Could you check a few things on this drawing? It's one solid part, dimensions in mm from its lowest x, y, z. Round coordinates to 2 decimals unless told otherwise and drop trailing zeros. Write each loop counter-clockwise with the first axis right and the second up, starting at its lowest first coordinate (ties: lowest second). Pieces come first, ordered by that corner, then holes. Notation, with made-up numbers: (2, 30.25) -> (37, 30.25) arc R20 cw to (37, 67.25) -> close; hole circle Ø8 at (-37, 68.25). An arc over 180 degrees is marked (long way). Answer in a Markdown table with one row per item. Add a question column.
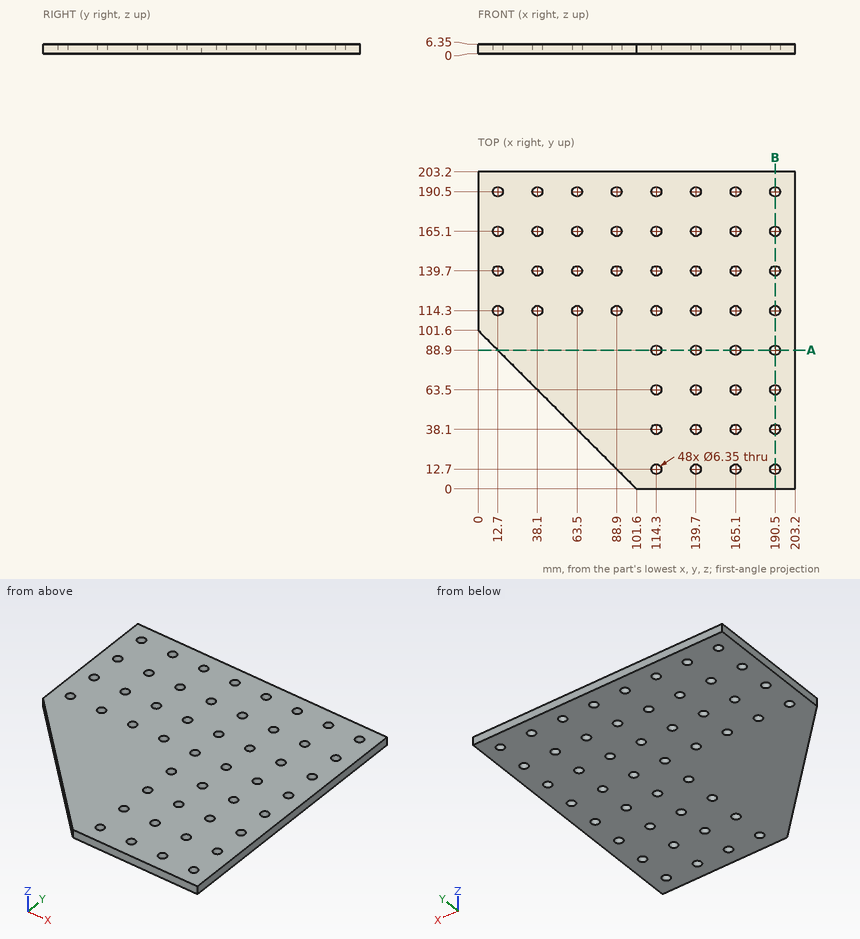
(1) For P1, Ø1, axis at y = 89, z = 5, coming from the -X side; P2, Ø8.5, axis at x = 165.1, y = 12.7, coming from the +Z side; P3, Ø2, axis at x = 28, z = 4.5, coming from the -Y side, each with a flat end and sliding along its axis, tell me the tip position at first contact or that it passes through.
(2) I need wall thicknesses on L1, parallel to Y at x = 12.7, z = 4 (3 decimals); L2, parallel to X at y = 37.5, z = 4.25; L3, parallel to Y at x = 91, z = 6. Which ranges of each line are inside material? Lowest first, please.
(3) Suppose I cut it at A-A, the plane y = 88.9. Please give me the cut outline in (x, z) (3 decimals).
(4) Suppose I cut it at B-B, the plane x = 190.5. State how many separate pieces and enclosed holes the cut face has, then the cut area to 3 significant figures.
Response:
| question | item | result |
|---|---|---|
| 1 | P1 | x = 12.1 |
| 1 | P2 | z = 6.35 |
| 1 | P3 | y = 72.6 |
| 2 | L1 | 88.9 to 111.125, 117.475 to 136.525, 142.875 to 161.925, 168.275 to 187.325, 193.675 to 203.2 |
| 2 | L2 | 64.1 to 111.18, 117.42 to 136.58, 142.82 to 161.98, 168.22 to 187.38, 193.62 to 203.2 |
| 2 | L3 | 10.6 to 111.92, 116.68 to 137.32, 142.08 to 162.72, 167.48 to 188.12, 192.88 to 203.2 |
| 3 | outline | (12.7, 0) -> (111.125, 0) -> (111.125, 6.35) -> (12.7, 6.35) -> close; (117.475, 0) -> (136.525, 0) -> (136.525, 6.35) -> (117.475, 6.35) -> close; (142.875, 0) -> (161.925, 0) -> (161.925, 6.35) -> (142.875, 6.35) -> close; (168.275, 0) -> (187.325, 0) -> (187.325, 6.35) -> (168.275, 6.35) -> close; (193.675, 0) -> (203.2, 0) -> (203.2, 6.35) -> (193.675, 6.35) -> close |
| 4 | separate pieces | 9 |
| 4 | enclosed holes | 0 |
| 4 | area | 968 mm² |
